```python
from build123d import *

# Parameters (mm, degrees)
SKETCH_1_R      = 1.5
EXTRUDE_1_DEPTH = 2
SKETCH_2_W      = 18.445036106
SKETCH_2_H      = 93.536016732
SKETCH_2_W_2    = 32.694926102
SKETCH_2_H_2    = 19.252727105
SKETCH_2_W_3    = 12.175605479
SKETCH_2_H_3    = 8.939965333
SKETCH_2_H_4    = 6.01746804
EXTRUDE_2_DEPTH = 15
SKETCH_3_W      = 17.224530095
SKETCH_3_H      = 17.900793214
EXTRUDE_3_DEPTH = 20


with BuildPart() as part:
    # 草图1 → 凸台-拉伸1 (new body)
    with BuildSketch(Plane.XY):
        Polygon((-66.211382114, 42.479674797), (-66.211382114, -47.520325203), (-66.211382114, -67.520325203), (11.788617886, -67.520325203), (26.788617886, -67.520325203), (26.788617886, 42.479674797), (26.788617886, 52.131300798), (-66.211382114, 52.131300798), align=None)
        with Locations((-38.211382114, 42.479674797)):
            Circle(SKETCH_1_R, mode=Mode.SUBTRACT)
        with Locations((11.788617886, 42.479674797)):
            Circle(SKETCH_1_R, mode=Mode.SUBTRACT)
        with Locations((11.788617886, -47.520325203)):
            Circle(SKETCH_1_R, mode=Mode.SUBTRACT)
        with Locations((-38.211382114, -47.520325203)):
            Circle(SKETCH_1_R, mode=Mode.SUBTRACT)
    extrude(amount=EXTRUDE_1_DEPTH)

    # 草图2 → 凸台-拉伸2 (add)
    with BuildSketch(Plane.XY.offset(2)):
        with Locations((-56.988864061, -3.180525851)):
            Rectangle(SKETCH_2_W, SKETCH_2_H)
        with Locations((-11.714742976, -57.893961651)):
            Rectangle(SKETCH_2_W_2, SKETCH_2_H_2)
        with Locations((20.700815147, -19.289017999)):
            Rectangle(SKETCH_2_W_3, SKETCH_2_H_3)
        with Locations((20.700815147, -40.681085502)):
            Rectangle(SKETCH_2_W_3, SKETCH_2_H_4)
    extrude(amount=EXTRUDE_2_DEPTH)

    # 草图3 → 凸台-拉伸3 (add)
    with BuildSketch(Plane.XY.offset(2)):
        with Locations((-33.897142446, -22.073097892)):
            Rectangle(SKETCH_3_W, SKETCH_3_H)
    extrude(amount=EXTRUDE_3_DEPTH)


solid = part.part
```
Design review of the part built by this model. Coordinates are the model's own, in mm. A direction names the side the tool comes from. Give positions to 0.01 mm unless a question says otherwise; leave off trailing zeros. Write each loop counter-clockwise with the first axis right and the second up, starting at its lowest first coordinate (ties: lowest second). Pieces come first, ordered by that corner, then holes. Notation, with made-up numbers: (40, -12) -> (45, -12) arc R20 cw to (45, 7) -> close; hole circle Ø9 at (39, -29.75). An arc over 180 degrees is marked (long way). Answer in a Markdown table with one row per item.
(1) Mouldability with a two-part tool opening along Y and no side actions: class faces 6 (the flat face through (21, -37.672, 9)), 7 (the flat face through (-57, 43.587, 9)), 8 (the cylindrical face through (-39.32, -46.51, 0.99)), 9 (the flat face through (-12, -58, 17)) as +Y half, -Y half, draft (parallel to the pull), parting line (faces both ways), or undercut.
Results:
| item | result |
|---|---|
| face 6 | undercut |
| face 7 | +Y half |
| face 8 | undercut |
| face 9 | draft |
(2) Consider section A-A (z = 8.5). State the section outline as (x, y) points, then the cut area to 3 significant figures.
Results:
| item | result |
|---|---|
| outline | (-66.21, -49.95) -> (-47.77, -49.95) -> (-47.77, 43.59) -> (-66.21, 43.59) -> close; (-42.51, -31.02) -> (-25.28, -31.02) -> (-25.28, -13.12) -> (-42.51, -13.12) -> close; (-28.06, -67.52) -> (4.63, -67.52) -> (4.63, -48.27) -> (-28.06, -48.27) -> close; (14.61, -43.69) -> (26.79, -43.69) -> (26.79, -37.67) -> (14.61, -37.67) -> close; (14.61, -23.76) -> (26.79, -23.76) -> (26.79, -14.82) -> (14.61, -14.82) -> close |
| area | 2,850 mm2 |
(3) Clearance check with flat-ended pins moving along their axes: pin 1 (8 mm diameter, centred on y = -12, z = 3.5, fed in from +X); pin 2 (1 mm diameter, centred on x = -55, z = 9, fed in from +Y); pin 3 (10 mm diameter, centred on x = 21.5, y = -17.5, fed in from +Z); pin 4 (10 mm diameter, centred on y = -4.5, z = 15, fed in from +X). State where each tip first meets the part, or that it passes through.
Results:
| item | result |
|---|---|
| pin 1 | x = 26.79 |
| pin 2 | y = 43.59 |
| pin 3 | z = 17 |
| pin 4 | x = -47.77 |
(4) Consider section C-C (y = -27.5). State the section outline as (x, z) points, then the cut area to 3 significant figures.
Results:
| item | result |
|---|---|
| outline | (-66.21, 0) -> (26.79, 0) -> (26.79, 2) -> (-25.28, 2) -> (-25.28, 22) -> (-42.51, 22) -> (-42.51, 2) -> (-47.77, 2) -> (-47.77, 17) -> (-66.21, 17) -> close |
| area | 807 mm2 |
(5) To check wall thickness, follow probe 1 along X at (y, z) = (-20, 15); probe 2 along Y at (x, z) = (20, 5.25); probe 3 along Y at (x, z) = (-25.5, 13). State the ranges of each line that lie inside material, in increasing order.
Results:
| item | result |
|---|---|
| probe 1 | -66.21 to -47.77, -42.51 to -25.28, 14.61 to 26.79 |
| probe 2 | -43.69 to -37.67, -23.76 to -14.82 |
| probe 3 | -67.52 to -48.27, -31.02 to -13.12 |
(6) For faces 1 (the flat face through (-34, -13.123, 12)), 2 (the flat face through (4.633, -58, 9)), 3 (the flat face through (14.613, -19, 9)), 4 (the flat face through (26.789, -21, 5)), 5 (the flat face through (-25.285, -22, 12)), list the 3-axis set-ups (+Z, -Z, +X, -X, +Y, -Y) from which the entire face can be reached by the end or side of a thin tool; tool diameter is ignored.
Results:
| item | result |
|---|---|
| face 1 | +Z, +X, +Y |
| face 2 | +Z, +X, +Y, -Y |
| face 3 | +Z, +Y, -Y |
| face 4 | +Z, -Z, +X, +Y, -Y |
| face 5 | +Z, +Y |
(7) Consider section B-B (x = 21). State the section outline as (y, z) points.
Results:
| item | result |
|---|---|
| outline | (-67.52, 0) -> (52.13, 0) -> (52.13, 2) -> (-14.82, 2) -> (-14.82, 17) -> (-23.76, 17) -> (-23.76, 2) -> (-37.67, 2) -> (-37.67, 17) -> (-43.69, 17) -> (-43.69, 2) -> (-67.52, 2) -> close |
(8) Consider section D-D (x = -38). State the section outline as (y, z) points.
Results:
| item | result |
|---|---|
| outline | (-67.52, 0) -> (-49.01, 0) -> (-49.01, 2) -> (-67.52, 2) -> close; (-46.04, 0) -> (40.99, 0) -> (40.99, 2) -> (-13.12, 2) -> (-13.12, 22) -> (-31.02, 22) -> (-31.02, 2) -> (-46.04, 2) -> close; (43.96, 0) -> (52.13, 0) -> (52.13, 2) -> (43.96, 2) -> close |
